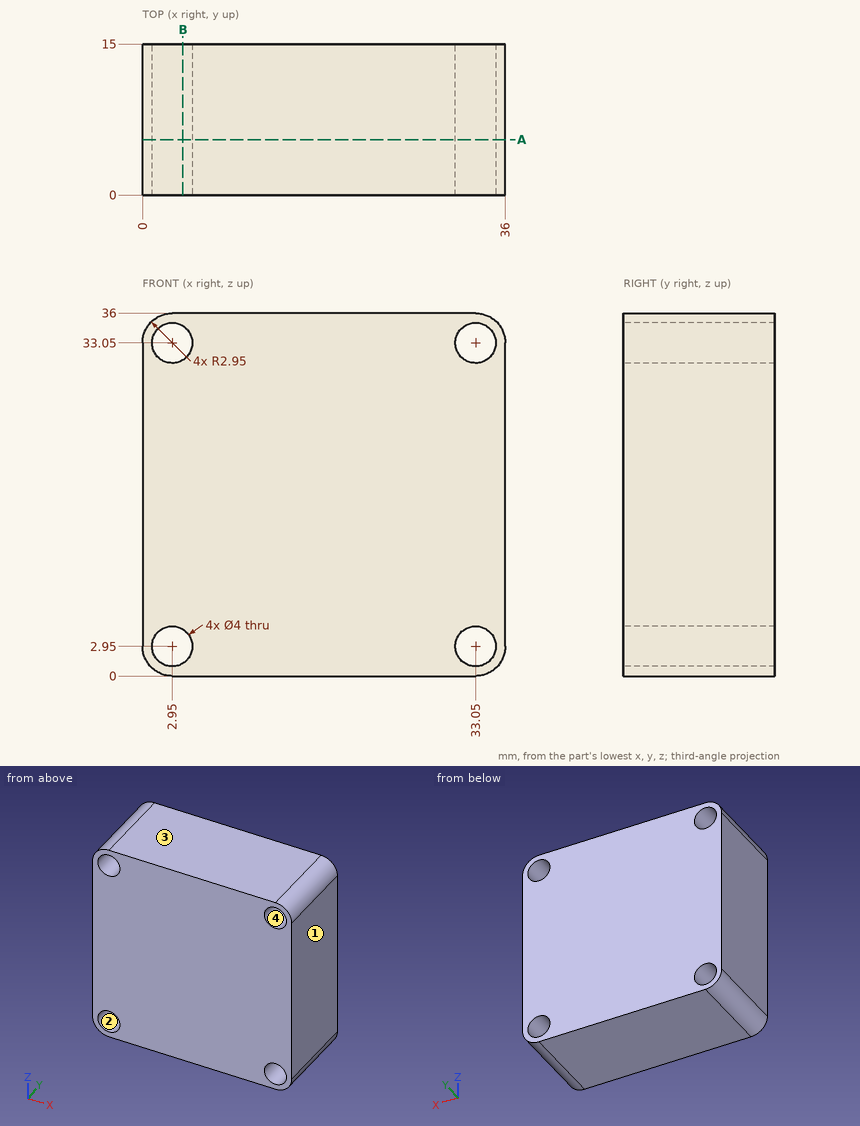
Here's the drawing with two shaded views (mm, measured from the low corner). I have some questions. Give positions to 0.01 mm unless a question says otherwise; leave off trailing zeros. Order: outer loops, then holes, each group sorted by start corner. A loop starts at its lowest first (then second) coordinate and runs counter-clockwise, first axis right, second up.
Q1. If I drill on line 1 along Z through (x, y) = (2.95, 6.5); line 2 along X through (y, z) = (8.25, 3.5); line 3 along Z through (x, y) = (4, 6.75), over which ranges is the centre line in solid material (lowest first)?
Q2. I'm going to push a flat-ended pin straight in: P1, Ø3.5, axis at x = 33.05, z = 33.05, coming from the +Y side. Where does the tip first touch, or does it pass through?
Q3. Suppose I cut it at A-A, the plane y = 5.5. Write out the boundary of the cut face in (x, z).
Q4. Suppose I cut it at B-B, the plane x = 4. Write out the boundary of the cut face in (y, z), and give its area (3 significant figures).
Q5. We'd pull the mould along Z, two halves only. Please class the marked faces 1, 2, 3 and 4: +Z half, -Z half, draft (parallel to the pull), parting line (faces both ways), or undercut.
Solution:
1. line 1: z = 0 to 0.95, 4.95 to 31.05, 35.05 to 36
1. line 2: x = 0 to 1.03, 4.87 to 31.13, 34.97 to 36
1. line 3: z = 0 to 1.25, 4.65 to 31.35, 34.75 to 36
2. P1: passes through
3. outline: (0, 2.95) arc R2.95 ccw to (2.95, 0) - (33.05, 0) arc R2.95 ccw to (36, 2.95) - (36, 33.05) arc R2.95 ccw to (33.05, 36) - (2.95, 36) arc R2.95 ccw to (0, 33.05) - close; hole circle Ø4 at (2.95, 2.95); hole circle Ø4 at (2.95, 33.05); hole circle Ø4 at (33.05, 2.95); hole circle Ø4 at (33.05, 33.05)
4. outline: (0, 0) - (15, 0) - (15, 1.25) - (0, 1.25) - close; (0, 4.65) - (15, 4.65) - (15, 31.35) - (0, 31.35) - close; (0, 34.75) - (15, 34.75) - (15, 36) - (0, 36) - close
4. area: 438 mm2
5. face 1: draft
5. face 2: undercut
5. face 3: +Z half
5. face 4: undercut
